Design review of the part built by this model. Coordinates are the model's own, in mm. Round coordinates to 2 decimals unless told otherwise and drop trailing zeros. Loops run counter-clockwise (first coordinate to the right, second up) from the corner with the lowest first, then second, coordinate; pieces in that order, holes last. Notation, with made-up numbers: (39.25, 24) - (69.25, 24) arc R25 cw to (69.25, 61) - close; hole circle Ø1 at (-28, -39). An arc over 180 degrees is marked (long way). Return JSON: item names as keys, results as strings. Group by question number.
(1) We need section A-A, the plane z = 3. Write out the cut boundary in (x, y), and give its area (3 significant figures).
(2) The part is to be moulded in two halves that separate along X. For faces 1 (the flat face through (0, -10, 3)), 2 (the cylindrical face through (9.867, -5.437, 3.67)), 3 (the flat face through (-12.5, -5, 3)), say which applies: pulls with the +X half, pulls with the -X half, needs draft (parallel to the pull), parting line crosses it, or undercut.
(3) Clearance check with a flat-ended pin moving along its axis: pin 1 (2 mm diameter, centred on x = -8.25, z = 3, fed in from +Y). State where the tip first meets the part, or that it passes through.
(4) We need section C-C, the plane x = -8.25. Write out the cut boundary in (y, z).
(5) We need section B-B, the plane y = -3. Write out the cut boundary in (x, z), and give its area (3 significant figures).
(6) Wall thickness on L1, parallel to X at y = -5.5, z = 3; L2, parallel to Z at x = 8.25, y = -3.25; L3, parallel to X at y = -2.25, z = 3.4: over which ranges is each line inside the solid? List them lowest first. Write a range as [from, to].
(7) We need section D-D, the plane y = -6. Write out the cut boundary in (x, z), and give its area (3 significant figures).
Autodesk Inventor part; units mm, degrees
ref_plane "YZ Plane" through (0, 0, 0) normal (1, 0, 0) x (0, 1, 0)
ref_plane "XZ Plane" through (0, 0, 0) normal (0, 1, 0) x (-1, 0, 0)
ref_plane "XY Plane" through (0, 0, 0) normal (0, 0, 1) x (1, 0, 0)
sketch "Sketch1" plane through (0, 0, 0) normal (0, 0, 1) x (1, 0, 0)
  arc A0 (-4, 0) -> (4, 0) centre (0, 0) ccw
  line L0 (-4, 0) -> (-12.5, 0)
  line L1 (-12.5, 0) -> (-12.5, -10)
  line L2 (-12.5, -10) -> (12.5, -10)
  line L3 (12.5, -10) -> (12.5, 0)
  line L4 (12.5, 0) -> (4, 0)
  dimension "d0" = 4
  dimension "d1" = 10
  dimension "d2" = 25
extrude "Extrusion1" add sketch "Sketch1" along normal blind 6
sketch "Sketch2" plane through (-12.5, 0, 0) normal (0, 1, 0) x (1, 0, 0)
  line L0 (0, 0) -> (8.5, 0)
  line L1 (8.5, -6) -> (0, -6)
  line L2 (16.5, 0) -> (25, 0)
  line L3 (16.5, 0) -> (16.5, -6)
  line L4 (25, -6) -> (16.5, -6)
  line L5 (25, 0) -> (25, -6)
  line L6 (4.25, 0) -> (4.25, -6) construction
  line L7 (20.75, 0) -> (20.75, -6) construction
  circle A0 centre (4.25, -3) radius 1.75
  circle A1 centre (20.75, -3) radius 1.75
  point P0 (12.5, 0)
  dimension "d5" = 3.5
extrude "Extrusion2" cut sketch "Sketch2" against normal through all contours A0 | A1
sketch "Sketch3" plane through (0, 0, 6) normal (0, 0, 1) x (1, 0, 0)
  line L0 (12.5, -10) -> (12.5, 0)
  line L1 (-12.5, 0) -> (12.5, 0)
  line L2 (12.5, 0) -> (12.5, -1)
  line L3 (12.5, -1) -> (-12.5, -1)
  line L4 (-12.5, -1) -> (-12.5, 0)
  dimension "d8" = 1
extrude "Extrusion3" cut sketch "Sketch3" against normal through all
properties part number "sensor bracket coupler"
Solutions:
{
 "1": {"outline": "(-12.5, -10) - (-10, -10) - (-10, -1) - (-12.5, -1) - close; (-6.5, -10) - (6.5, -10) - (6.5, -1) - (3.87, -1) arc R4 cw to (-3.87, -1) - (-6.5, -1) - close; (10, -10) - (12.5, -10) - (12.5, -1) - (10, -1) - close", "area": "145 mm^2"},
 "2": {"face 1": "needs draft", "face 2": "undercut", "face 3": "pulls with the -X half"},
 "3": {"pin 1": "through"},
 "4": {"outline": "(-10, 0) - (-1, 0) - (-1, 1.25) - (-10, 1.25) - close; (-10, 4.75) - (-1, 4.75) - (-1, 6) - (-10, 6) - close"},
 "5": {"outline": "(-12.5, 0) - (-2.65, 0) - (-2.65, 6) - (-12.5, 6) - close; (2.65, 0) - (12.5, 0) - (12.5, 6) - (2.65, 6) - close; hole circle Ø3.5 at (-8.25, 3); hole circle Ø3.5 at (8.25, 3)", "area": "99.0 mm^2"},
 "6": {"L1": "[-12.5, -10], [-6.5, 6.5], [10, 12.5]", "L2": "[0, 1.25], [4.75, 6]", "L3": "[-12.5, -9.95], [-6.55, -3.31], [3.31, 6.55], [9.95, 12.5]"},
 "7": {"outline": "(-12.5, 0) - (12.5, 0) - (12.5, 6) - (-12.5, 6) - close; hole circle Ø3.5 at (-8.25, 3); hole circle Ø3.5 at (8.25, 3)", "area": "131 mm^2"}
}
